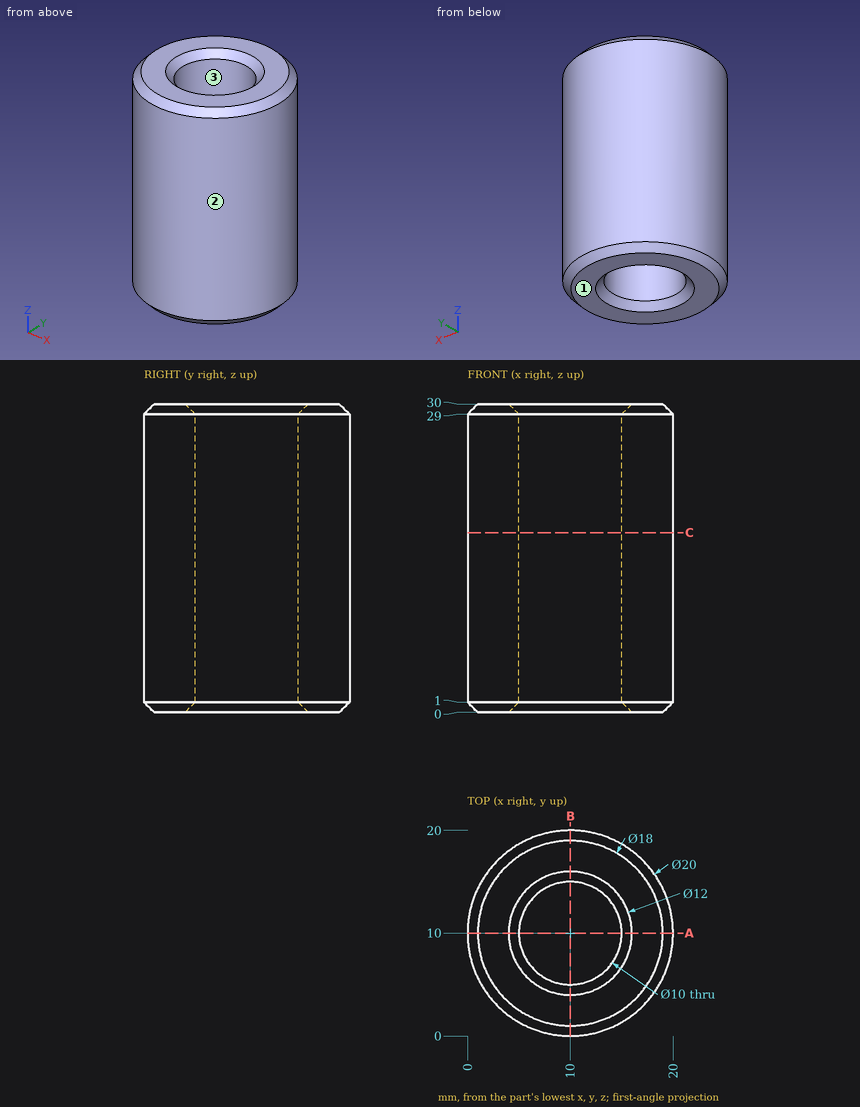
Job drawing, mm, ordinate dimensions from the low corner. One solid piece. Round coordinates to 2 decimals unless told otherwise and drop trailing zeros. Write each loop counter-clockwise with the first axis right and the second up, starting at its lowest first coordinate (ties: lowest second). Pieces come first, ordered by that corner, then holes. Notation, with made-up numbers: (81, 69) -> (105, 69) arc R33 ccw to (105, 97) -> close; hole circle Ø7 at (35.5, 75.25). An arc over 180 degrees is marked (long way). Answer as CSV lines item,"result".
1. Drill centre lines: line 1 (Y direction, x = 9.75, z = 17.25); line 2 (Y direction, x = 11, z = 9); line 3 (X direction, y = 8.5, z = 10.5). Where is each one in solid material? Low to high.
Resolved:
line 1,"0 to 5.01, 14.99 to 20"
line 2,"0.05 to 5.1, 14.9 to 19.95"
line 3,"0.11 to 5.23, 14.77 to 19.89"
2. Slice it at C-C, the plane z = 17.5. List the corners of the cut face in (x, y), plus the area to 3 significant figures.
Resolved:
outline,"circle Ø20 at (10, 10); hole circle Ø10 at (10, 10)"
area,"236 mm²"
3. Mould opens along X. For the marked faces 1, 2 and 3 say: +X half, -X half, draft (parallel to the pull), parting line (faces both ways), or undercut.
Resolved:
face 1,"draft"
face 2,"parting line"
face 3,"undercut"
4. Pin check, flat tips, straight feed: pin 1 Ø2 at (y, z) = (12.5, 14.5) entering from +X; pin 2 Ø2 at (x, y) = (14, 7.5) entering from -Z; pin 3 Ø1 at (x, z) = (15.5, 14.5) entering from -Y. Stop position of each tip, or through.
Resolved:
pin 1,"x = 19.89"
pin 2,"z = 0.28"
pin 3,"y = 1.34"
5. Slice it at A-A, the plane y = 10. List the corners of the cut face in (x, z), plus the area to 3 significant figures.
Resolved:
outline,"(0, 1) -> (1, 0) -> (4, 0) -> (5, 1) -> (5, 29) -> (4, 30) -> (1, 30) -> (0, 29) -> close; (15, 1) -> (16, 0) -> (19, 0) -> (20, 1) -> (20, 29) -> (19, 30) -> (16, 30) -> (15, 29) -> close"
area,"296 mm²"
